from build123d import *

# Parameters (mm, degrees)
F0_W     = 427.5
F0_H     = 30
F0_W_2   = 30
F0_H_2   = 427.5
F1_DEPTH = 350
F3_DEPTH = 22


with BuildPart() as f1:
    # F0 (on Front) → F1 (new body)
    with BuildSketch(Plane.XZ):
        with BuildLine():
            Line((386.3346025348, 1120.6153738732), (-1413.6653974652, 1120.6153738732))
            ThreePointArc((-1413.6653974652, 1120.6153738732), (-1484.3760755839, 1091.3260519918), (-1513.6653974652, 1020.6153738732))
            Line((-1513.6653974652, 1020.6153738732), (-1513.6653974652, -779.3846261268))
            ThreePointArc((-1513.6653974652, -779.3846261268), (-1484.3760755839, -850.0953042455), (-1413.6653974652, -879.3846261268))
            Line((-1413.6653974652, -879.3846261268), (386.3346025348, -879.3846261268))
            ThreePointArc((386.3346025348, -879.3846261268), (457.0452806534, -850.0953042455), (486.3346025348, -779.3846261268))
            Line((486.3346025348, -779.3846261268), (486.3346025348, 1020.6153738732))
            ThreePointArc((486.3346025348, 1020.6153738732), (457.0452806534, 1091.3260519918), (386.3346025348, 1120.6153738732))
        make_face()
        with BuildLine():
            ThreePointArc((-1413.6653974652, 920.6153738732), (-1384.3760755839, 991.3260519918), (-1313.6653974652, 1020.6153738732))
            Line((-1313.6653974652, 1020.6153738732), (-986.1653974652, 1020.6153738732))
            Line((-986.1653974652, 1020.6153738732), (-956.1653974652, 1020.6153738732))
            Line((-956.1653974652, 1020.6153738732), (-528.6653974652, 1020.6153738732))
            Line((-528.6653974652, 1020.6153738732), (-498.6653974652, 1020.6153738732))
            Line((-498.6653974652, 1020.6153738732), (-71.1653974652, 1020.6153738732))
            Line((-71.1653974652, 1020.6153738732), (-41.1653974652, 1020.6153738732))
            Line((-41.1653974652, 1020.6153738732), (286.3346025348, 1020.6153738732))
            ThreePointArc((286.3346025348, 1020.6153738732), (357.0452806534, 991.3260519918), (386.3346025348, 920.6153738732))
            Line((386.3346025348, 920.6153738732), (386.3346025348, 593.1153738732))
            Line((386.3346025348, 593.1153738732), (386.3346025348, 563.1153738732))
            Line((386.3346025348, 563.1153738732), (386.3346025348, 135.6153738732))
            Line((386.3346025348, 135.6153738732), (386.3346025348, 105.6153738732))
            Line((386.3346025348, 105.6153738732), (386.3346025348, -321.8846261268))
            Line((386.3346025348, -321.8846261268), (386.3346025348, -351.8846261268))
            Line((386.3346025348, -351.8846261268), (386.3346025348, -679.3846261268))
            ThreePointArc((386.3346025348, -679.3846261268), (357.0452806534, -750.0953042455), (286.3346025348, -779.3846261268))
            Line((286.3346025348, -779.3846261268), (-41.1653974652, -779.3846261268))
            Line((-41.1653974652, -779.3846261268), (-71.1653974652, -779.3846261268))
            Line((-71.1653974652, -779.3846261268), (-498.6653974652, -779.3846261268))
            Line((-498.6653974652, -779.3846261268), (-528.6653974652, -779.3846261268))
            Line((-528.6653974652, -779.3846261268), (-956.1653974652, -779.3846261268))
            Line((-956.1653974652, -779.3846261268), (-986.1653974652, -779.3846261268))
            Line((-986.1653974652, -779.3846261268), (-1313.6653974652, -779.3846261268))
            ThreePointArc((-1313.6653974652, -779.3846261268), (-1384.3760755839, -750.0953042455), (-1413.6653974652, -679.3846261268))
            Line((-1413.6653974652, -679.3846261268), (-1413.6653974652, -351.8846261268))
            Line((-1413.6653974652, -351.8846261268), (-1413.6653974652, -321.8846261268))
            Line((-1413.6653974652, -321.8846261268), (-1413.6653974652, 105.6153738732))
            Line((-1413.6653974652, 105.6153738732), (-1413.6653974652, 135.6153738732))
            Line((-1413.6653974652, 135.6153738732), (-1413.6653974652, 563.1153738732))
            Line((-1413.6653974652, 563.1153738732), (-1413.6653974652, 593.1153738732))
            Line((-1413.6653974652, 593.1153738732), (-1413.6653974652, 920.6153738732))
        make_face(mode=Mode.SUBTRACT)
        with Locations((-742.4153974652, 578.1153738732)):
            Rectangle(F0_W, F0_H)
        with Locations((-1199.9153974652, 578.1153738732)):
            Rectangle(F0_W, F0_H)
        with Locations((-971.1653974652, 806.8653738732)):
            Rectangle(F0_W_2, F0_H_2)
        with Locations((-971.1653974652, 578.1153738732)):
            Rectangle(F0_W_2, F0_H)
        with Locations((-513.6653974652, 806.8653738732)):
            Rectangle(F0_W_2, F0_H_2)
        with Locations((-513.6653974652, 578.1153738732)):
            Rectangle(F0_W_2, F0_H)
        with Locations((-284.9153974652, 578.1153738732)):
            Rectangle(F0_W, F0_H)
        with Locations((-56.1653974652, 806.8653738732)):
            Rectangle(F0_W_2, F0_H_2)
        with Locations((-56.1653974652, 578.1153738732)):
            Rectangle(F0_W_2, F0_H)
        with Locations((172.5846025348, 578.1153738732)):
            Rectangle(F0_W, F0_H)
        with Locations((-56.1653974652, 349.3653738732)):
            Rectangle(F0_W_2, F0_H_2)
        with Locations((-513.6653974652, 349.3653738732)):
            Rectangle(F0_W_2, F0_H_2)
        with Locations((-971.1653974652, 349.3653738732)):
            Rectangle(F0_W_2, F0_H_2)
        with Locations((-1199.9153974652, 120.6153738732)):
            Rectangle(F0_W, F0_H)
        with Locations((-971.1653974652, 120.6153738732)):
            Rectangle(F0_W_2, F0_H)
        with Locations((-742.4153974652, 120.6153738732)):
            Rectangle(F0_W, F0_H)
        with Locations((-284.9153974652, 120.6153738732)):
            Rectangle(F0_W, F0_H)
        with Locations((-513.6653974652, 120.6153738732)):
            Rectangle(F0_W_2, F0_H)
        with Locations((-56.1653974652, 120.6153738732)):
            Rectangle(F0_W_2, F0_H)
        with Locations((172.5846025348, 120.6153738732)):
            Rectangle(F0_W, F0_H)
        with Locations((-56.1653974652, -336.8846261268)):
            Rectangle(F0_W_2, F0_H)
        with Locations((-513.6653974652, -336.8846261268)):
            Rectangle(F0_W_2, F0_H)
        with Locations((-971.1653974652, -336.8846261268)):
            Rectangle(F0_W_2, F0_H)
        with Locations((-971.1653974652, -108.1346261268)):
            Rectangle(F0_W_2, F0_H_2)
        with Locations((-513.6653974652, -108.1346261268)):
            Rectangle(F0_W_2, F0_H_2)
        with Locations((-742.4153974652, -336.8846261268)):
            Rectangle(F0_W, F0_H)
        with Locations((-284.9153974652, -336.8846261268)):
            Rectangle(F0_W, F0_H)
        with Locations((172.5846025348, -336.8846261268)):
            Rectangle(F0_W, F0_H)
        with Locations((-56.1653974652, -108.1346261268)):
            Rectangle(F0_W_2, F0_H_2)
        with Locations((-56.1653974652, -565.6346261268)):
            Rectangle(F0_W_2, F0_H_2)
        with Locations((-513.6653974652, -565.6346261268)):
            Rectangle(F0_W_2, F0_H_2)
        with Locations((-971.1653974652, -565.6346261268)):
            Rectangle(F0_W_2, F0_H_2)
        with Locations((-1199.9153974652, -336.8846261268)):
            Rectangle(F0_W, F0_H)
    extrude(amount=F1_DEPTH)

    # F2 (on face) → F3 (join)
    with BuildSketch(Plane(origin=(0, 0, 0), x_dir=(-1, 0, 0), z_dir=(0, 1, 0))):
        with BuildLine():
            Line((1418.2799100876, 1120.6153738732), (-386.3346025348, 1120.6153738732))
            ThreePointArc((-386.3346025348, 1120.6153738732), (-457.0452806534, 1091.3260519918), (-486.3346025348, 1020.6153738732))
            Line((-486.3346025348, 1020.6153738732), (-486.3346025348, -781.5458416939))
            ThreePointArc((-486.3346025348, -781.5458416939), (-457.0452806534, -852.2565198125), (-386.3346025348, -881.5458416939))
            Line((-386.3346025348, -881.5458416939), (1418.2799100876, -881.5458416939))
            ThreePointArc((1418.2799100876, -881.5458416939), (1488.9905882062, -852.2565198125), (1518.2799100876, -781.5458416939))
            Line((1518.2799100876, -781.5458416939), (1518.2799100876, 1020.6153738732))
            ThreePointArc((1518.2799100876, 1020.6153738732), (1488.9905882062, 1091.3260519918), (1418.2799100876, 1120.6153738732))
        make_face()
    extrude(amount=F3_DEPTH)


solid = f1.part
Build history of the part. All positions in model axes, mm. Round coordinates to 2 decimals unless told otherwise and drop trailing zeros. Write each loop counter-clockwise with the first axis right and the second up, starting at its lowest first coordinate (ties: lowest second). Pieces come first, ordered by that corner, then holes. Notation, with made-up numbers: M -21,8.25 L -12,8.25 A23 ccw -12,24.25 Z; hole C 80,44 d5. An arc over 180 degrees is marked long. Answer in a Markdown table with one row per item.
1. Saw through at C-C (y = -25). State how many separate pieces and enclosed holes the cut face has, and give its area (3 significant figures).
Geometry check:
| item | result |
|---|---|
| separate pieces | 1 |
| enclosed holes | 16 |
| area | 1,080,000 mm2 |
2. Flat gauge pins, fed straight in: P1, Ø2, axis at x = -557.5, y = -273, coming from the -Z side; P2, Ø1.5, axis at x = 216.5, z = -471.5, coming from the -Y side. Where does each tip first touch, or does it go through?
Geometry check:
| item | result |
|---|---|
| P1 | z = -879.38 |
| P2 | y = 0 |
3. Probe L1, parallel to X at y = -78, z = 29; L2, parallel to Z at x = -244.5, y = -171; L3, parallel to Z at x = -1397, y = -57.5. List the from-to ranges inside material, lowest first. Write a range as [from, to].
Geometry check:
| item | result |
|---|---|
| L1 | [-1513.67, -1413.67], [-986.17, -956.17], [-528.67, -498.67], [-71.17, -41.17], [386.33, 486.33] |
| L2 | [-879.38, -779.38], [-351.88, -321.88], [105.62, 135.62], [563.12, 593.12], [1020.62, 1120.62] |
| L3 | [-879.38, -734.66], [-351.88, -321.88], [105.62, 135.62], [563.12, 593.12], [975.89, 1120.62] |
4. Mould opens along Z. For faces 1 (the face through (486.335, -167, 132)), 2 (the face through (456.26, -166.6, 1092.1)), 3 (the face through (-986.165, -173, 346)) say: +Z half, -Z half, draft (parallel to the pull), parting line (faces both ways), or undercut.
Geometry check:
| item | result |
|---|---|
| face 1 | draft |
| face 2 | +Z half |
| face 3 | undercut |
5. Saw through at B-B (x = -346). List the corners of the cut face in (y, z), and give its area (3 significant figures).
Geometry check:
| item | result |
|---|---|
| outline | M -350,-879.38 L 0,-879.38 L 0,-881.55 L 22,-881.55 L 22,1120.62 L -350,1120.62 L -350,1020.62 L 0,1020.62 L 0,593.12 L -350,593.12 L -350,563.12 L 0,563.12 L 0,135.62 L -350,135.62 L -350,105.62 L 0,105.62 L 0,-321.88 L -350,-321.88 L -350,-351.88 L 0,-351.88 L 0,-779.38 L -350,-779.38 Z |
| area | 146,000 mm2 |
6. Saw through at A-A (z = -563). List the corners of the cut face in (x, y), and give its area (3 significant figures).
Geometry check:
| item | result |
|---|---|
| outline | M -1518.28,0 L -1513.67,0 L -1513.67,-350 L -1413.67,-350 L -1413.67,0 L -986.17,0 L -986.17,-350 L -956.17,-350 L -956.17,0 L -528.67,0 L -528.67,-350 L -498.67,-350 L -498.67,0 L -71.17,0 L -71.17,-350 L -41.17,-350 L -41.17,0 L 386.33,0 L 386.33,-350 L 486.33,-350 L 486.33,22 L -1518.28,22 Z |
| area | 146,000 mm2 |
